Build history of the part. All positions in model axes, mm. Face numbers are marked on the shaded views. A direction names the side the tool comes from. Round coordinates to 2 decimals unless told otherwise and drop trailing zeros. Write each loop counter-clockwise with the first axis right and the second up, starting at its lowest first coordinate (ties: lowest second). Pieces come first, ordered by that corner, then holes. Notation, with made-up numbers: (-21, 19.25) - (-2, 19.25) arc R21 cw to (-2, 39.25) - close; hole circle Ø6 at (35, -22.75). An arc over 180 degrees is marked (long way). One line per question, with ' | ' between items.
from build123d import *

# Parameters (mm, degrees)
F1_DEPTH     = 9
F2_R         = 2
F3_R         = 3
F3_R_2       = 2
F4_DEPTH     = 18
F5_R         = 7
F6_DEPTH     = 5
F8_R         = 7.5
F9_DEPTH     = 5
F10_S5_R     = 7
F10_T6_DEPTH = 12
F11_R        = 7
F12_DEPTH    = 2
F13_SIZE     = 1
F14_R        = 4.5
F15_DEPTH    = 1.5
F16_R        = 3
F17_DEPTH    = 15
F18_R        = 7
F19_DEPTH    = 5
F20_R        = 7.5
F21_DEPTH    = 5
F22_R        = 7
F23_DEPTH    = 2
F24_R        = 4.5
F25_DEPTH    = 1.5
F26_R        = 3
F27_DEPTH    = 25
F28_S7_R     = 7
F28_T8_DEPTH = 12


# Not quite as in the source:
# - a fillet or chamfer that OpenCascade refuses, or shapes differently, is made with other operations: its cross-section is extruded or revolved along the edge and cut away or added
# - a feature names something its author has since deleted; it is built from what else it names


with BuildPart() as f1:
    # F0 (on Top) → F1 (new body)
    with BuildSketch(Plane.XY):
        Polygon((-10, -4.5), (3, -4.5), (3, 4.5), (0, 4.5), (0, 6.5), (-9, 6.5), (-9, 4.5), (-10, 4.5), align=None)
    extrude(amount=F1_DEPTH)

    # F2
    f2_edges = [f1.edges().sort_by_distance(p)[0] for p in [
        (-3.5, -4.5, 9),
        (-3.5, -4.5, 0),
        (1.5, 4.5, 0),
        (1.5, 4.5, 9),
        (-9.5, 4.5, 9),
        (-9.5, 4.5, 0),
    ]]
    fillet(f2_edges, radius=F2_R)

    # F3 (on face) → F4 (join)
    with BuildSketch(Plane(origin=(-10, 0, 0), x_dir=(0, -1, 0), z_dir=(-1, 0, 0))):
        with Locations((0, 4.5)):
            Circle(F3_R)
        with Locations((0, 4.5)):
            Circle(F3_R_2, mode=Mode.SUBTRACT)
    extrude(amount=F4_DEPTH)

    # F5 (on face) → F6 (join)
    with BuildSketch(Plane(origin=(0, 6.5, 0), x_dir=(-1, 0, 0), z_dir=(0, 1, 0))):
        with Locations((4.5, 4.5)):
            Circle(F5_R)
    extrude(amount=F6_DEPTH)

    # F7: chamfer of 1 on 1 edges, made by hand


with BuildPart() as f7_tool2:
    # F7_s3 → F7_t4 (revolve)
    with BuildSketch(Plane.XY.offset(4.5)):
        Polygon((-11.5, 7.5), (-10.5, 6.5), (-11.5, 6.5), align=None)
    revolve(axis=Axis((-4.5, 6.5, 4.5), (0, 1, 0)))

    split(bisect_by=Plane.YZ.offset(-9), keep=Keep.BOTTOM)


with BuildPart() as f1_1:
    add(f1.part)

    # F7_t1: cut F7_tool2
    add(f7_tool2.part, mode=Mode.SUBTRACT)


with BuildPart() as f7_tool7:
    # F7_s8 → F7_t9 (revolve)
    with BuildSketch(Plane.XY.offset(4.5)):
        Polygon((-11.5, 7.5), (-10.5, 6.5), (-11.5, 6.5), align=None)
    revolve(axis=Axis((-4.5, 6.5, 4.5), (0, 1, 0)))

    split(bisect_by=Plane.XY.offset(9), keep=Keep.TOP)


with BuildPart() as f1_2:
    add(f1_1.part)

    # F7_t6: cut F7_tool7
    add(f7_tool7.part, mode=Mode.SUBTRACT)


with BuildPart() as f7_tool12:
    # F7_s13 → F7_t14 (revolve)
    with BuildSketch(Plane.XY.offset(4.5)):
        Polygon((-11.5, 7.5), (-10.5, 6.5), (-11.5, 6.5), align=None)
    revolve(axis=Axis((-4.5, 6.5, 4.5), (0, 1, 0)))

    split(bisect_by=Plane.XY, keep=Keep.BOTTOM)


with BuildPart() as f1_3:
    add(f1_2.part)

    # F7_t11: cut F7_tool12
    add(f7_tool12.part, mode=Mode.SUBTRACT)


with BuildPart() as f7_tool17:
    # F7_s18 → F7_t19 (revolve)
    with BuildSketch(Plane.XY.offset(4.5)):
        Polygon((-11.5, 7.5), (-10.5, 6.5), (-11.5, 6.5), align=None)
    revolve(axis=Axis((-4.5, 6.5, 4.5), (0, 1, 0)))

    split(bisect_by=Plane.YZ, keep=Keep.TOP)


with BuildPart() as f1_4:
    add(f1_3.part)

    # F7_t16: cut F7_tool17
    add(f7_tool17.part, mode=Mode.SUBTRACT)

    # F8 (on face) → F9 (join)
    with BuildSketch(Plane(origin=(0, 11.5, 0), x_dir=(-1, 0, 0), z_dir=(0, 1, 0))):
        with Locations((4.5, 4.5)):
            Circle(F8_R)
    extrude(amount=F9_DEPTH)

    # F10: chamfer of 1 on 1 edges, made by hand


with BuildPart() as f10_tool2:
    # F10_s3 → F10_t4 (revolve)
    with BuildSketch(Plane.XY.offset(4.5)):
        Polygon((-12, 12.5), (-11, 11.5), (-12, 11.5), align=None)
    revolve(axis=Axis((-4.5, 11.5, 4.5), (0, 1, 0)))

    # F10_s5 → F10_t6 (cut, symmetric)
    with BuildSketch(Plane.XZ.offset(-12)):
        with Locations((-4.5, 4.5)):
            Circle(F10_S5_R)
    extrude(amount=F10_T6_DEPTH, both=True, mode=Mode.SUBTRACT)


with BuildPart() as f1_5:
    add(f1_4.part)

    # F10_t1: cut F10_tool2
    add(f10_tool2.part, mode=Mode.SUBTRACT)

    # F11 (on face) → F12 (join)
    with BuildSketch(Plane(origin=(0, 16.5, 0), x_dir=(-1, 0, 0), z_dir=(0, 1, 0))):
        with Locations((4.5, 4.5)):
            Circle(F11_R)
    extrude(amount=F12_DEPTH)

    # F13
    f13_edges = [f1_5.edges().sort_by_distance(p)[0] for p in [
        (2.5, 18.5, 4.5),
    ]]
    chamfer(f13_edges, length=F13_SIZE)

    # F14 (on face) → F15 (join)
    with BuildSketch(Plane(origin=(0, 18.5, 0), x_dir=(-1, 0, 0), z_dir=(0, 1, 0))):
        with Locations((4.5, 4.5)):
            Circle(F14_R)
    extrude(amount=F15_DEPTH)

    # F16 (on face) → F17 (cut)
    with BuildSketch(Plane(origin=(0, 20, 0), x_dir=(-1, 0, 0), z_dir=(0, 1, 0))):
        with Locations((4.5, 4.5)):
            Circle(F16_R)
    extrude(amount=-F17_DEPTH, mode=Mode.SUBTRACT)

    # F18 (on face) → F19 (join)
    with BuildSketch(Plane.YZ.offset(3)):
        with Locations((0, 4.5)):
            Circle(F18_R)
    extrude(amount=F19_DEPTH)

    # F20 (on face) → F21 (join)
    with BuildSketch(Plane.YZ.offset(8)):
        with Locations((0, 4.5)):
            Circle(F20_R)
    extrude(amount=F21_DEPTH)

    # F22 (on face) → F23 (join)
    with BuildSketch(Plane.YZ.offset(13)):
        with Locations((0, 4.5)):
            Circle(F22_R)
    extrude(amount=F23_DEPTH)

    # F24 (on face) → F25 (join)
    with BuildSketch(Plane.YZ.offset(15)):
        with Locations((0, 4.5)):
            Circle(F24_R)
    extrude(amount=F25_DEPTH)

    # F26 (on face) → F27 (cut)
    with BuildSketch(Plane.YZ.offset(16.5)):
        with Locations((0, 4.5)):
            Circle(F26_R)
    extrude(amount=-F27_DEPTH, mode=Mode.SUBTRACT)

    # F28: chamfer of 1 on 3 edges, made by hand

    # F28_s1 → F28_t2 (revolve, cut)
    with BuildSketch(Plane.XY.offset(4.5)):
        Polygon((4, 7), (3, 6), (3, 7), align=None)
    revolve(axis=Axis((3, 0, 4.5), (1, 0, 0)), mode=Mode.SUBTRACT)


with BuildPart() as f28_tool4:
    # F28_s5 → F28_t6 (revolve)
    with BuildSketch(Plane.XY.offset(4.5)):
        Polygon((9, 7.5), (8, 6.5), (8, 7.5), align=None)
    revolve(axis=Axis((8, 0, 4.5), (1, 0, 0)))

    # F28_s7 → F28_t8 (cut, symmetric)
    with BuildSketch(Plane.YZ.offset(8.5)):
        with Locations((0, 4.5)):
            Circle(F28_S7_R)
    extrude(amount=F28_T8_DEPTH, both=True, mode=Mode.SUBTRACT)


with BuildPart() as f1_6:
    add(f1_5.part)

    # F28_t3: cut F28_tool4
    add(f28_tool4.part, mode=Mode.SUBTRACT)

    # F28_s9 → F28_t10 (revolve, cut)
    with BuildSketch(Plane.XY.offset(4.5)):
        Polygon((14, 7), (15, 6), (15, 7), align=None)
    revolve(axis=Axis((15, 0, 4.5), (1, 0, 0)), mode=Mode.SUBTRACT)


solid = f1_6.part
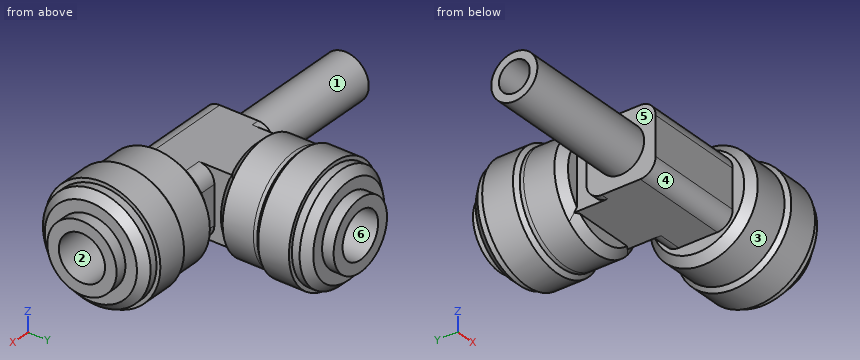
Q1. Drill centre lines: L1, parallel to X at y = 6, z = 6.5; L2, parallel to Z at x = -4.5, y = 8; L3, parallel to Z at x = -4.5, y = 12.75. Where is each one in solid material? Low to high. Write a range as from..to.
Found:
L1: -9..-6.74, -2.26..0, 3.32..14.68 | L2: -2.5..1.5, 7.5..11.5 | L3: -3..1.5, 7.5..12
Q2. Which spindle directions (+Z, -Z, +X, -X, +Y, -Y) get a long thin tool onto all of the face, cutting with end or side? Do the marked faces 1, 2 and 3. Say none if no direction does.
Found:
face 1: -X | face 2: +X | face 3: none
Q3. Saw through at C-C, the plane x = -18. List the corners of the cut face in (y, z).
Found:
outline: circle Ø6 at (0, 4.5); hole circle Ø4 at (0, 4.5)
Q4. Pull direction X, two halves, no side cores. Call the marked faces 4, 5 and 6: +X half, -X half, draft (parallel to the pull), parting line (faces both ways), or undercut.
Found:
face 4: draft | face 5: -X half | face 6: undercut
Q5. Saw through at B-B, the plane y = 10.5. List the corners of the cut face in (x, z), then the cut area to 3 significant figures.
Found:
outline: circle Ø14 at (-4.5, 4.5); hole circle Ø6 at (-4.5, 4.5) | area: 126 mm^2
Q6. Drop flat-ended pins along their axis: pin 1 (3 mm diameter, centred on x = -4.5, y = -1, fed in from -Z); pin 2 (10.5 mm diameter, centred on x = -0.5, y = 2.5, fed in from -Z); pin 3 (4 mm diameter, centred on x = -23, y = 4, fed in from -Z). Give the stop position or say it passes through.
Found:
pin 1: z = 0 | pin 2: z = -2.5 | pin 3: z = 2.26
